Source: CAD feature listing. Evaluate the final solid. Frame: model axes, mm. Face numbers are marked on the shaded views. A direction names the side the tool comes from. Give positions to 0.01 mm unless a question says otherwise; leave off trailing zeros. Order: outer loops, then holes, each group sorted by start corner. A loop starts at its lowest first (then second) coordinate and runs counter-clockwise, first axis right, second up. Notation, with made-up numbers: (10, 18) - (14, 18) arc R34 ccw to (14, 49) - close; hole circle Ø11 at (22, 44.25). An arc over 180 degrees is marked (long way). Write each question's results on one line, items separated by ' | '. Start each with the question number.
Item 1: Line query: line 1 along X through (y, z) = (-12.75, 5.25); line 2 along Z through (x, y) = (12, -10); line 3 along Y through (x, z) = (5, 1.15). Output: solid intervals per line, ascending.
Item 2: Mould query, pull axis X, two halves, no side actions, for the marked faces 4, 5 and 6. Classes: released by +X, released by -X, zero draft, split by the parting line, or undercut.
Item 3: Section D-D on x = 31.5. Output: boundary loops of the cut face in (y, z) (1 decimal), and give its area (3 significant figures).
Item 4: Section A-A on x = 4.5. Output: boundary loops of the cut face in (y, z).
Item 5: Contact query for flat-ended pins moving along their axis: pin 1 Ø6 at (x, y) = (6, -4) entering from -Z; pin 2 Ø1.3 at (x, y) = (14.5, -6.5) entering from +Z; pin 3 Ø1.4 at (x, z) = (23, 12.5) entering from +Y; pin 4 Ø2 at (x, z) = (23.5, 11) entering from -Y. Output: stop coordinate, or through.
Item 6: Set-up query: the marked faces 1, 2 and 3. Return all of +Z, -Z, +X, -X, +Y, -Y with unobstructed straight access to the full face (end or side cutting, diameter ignored); none if empty.
Item 7: Section B-B on y = -10. State how many separate pieces and enclosed holes the cut face has, and give its area (3 significant figures).
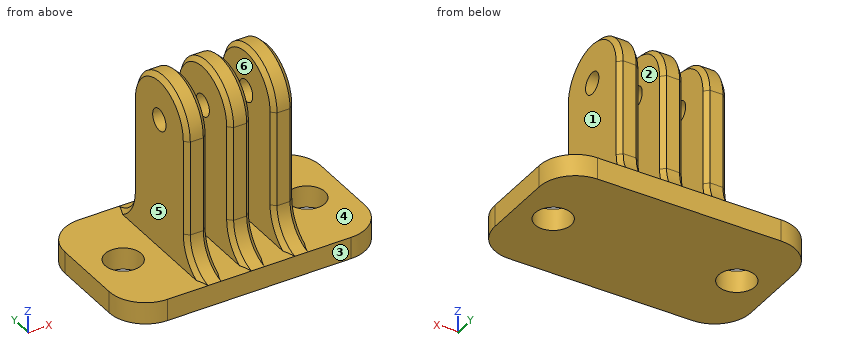
```python
from build123d import *

# Parameters (mm, degrees)
SKETCH_1_W             = 35.4
SKETCH_1_H             = 20
SKETCH_1_R             = 2.5
EXTRUDE_1_DEPTH        = 3
EXTRUDE_START          = -10
SKETCH_3_R             = 1.5
EXTRUDE_2_DEPTH        = 3
PATTERN_LINEAR_1_COUNT = 3
PATTERN_LINEAR_1_PITCH = 6
FILLET_1_R             = 5
CHAMFER_1_SIZE         = 0.6


with BuildPart() as part:
    # 草图1 → 凸台-拉伸1 (new body)
    with BuildSketch(Plane.XY):
        with Locations((17.7, -10)):
            Rectangle(SKETCH_1_W, SKETCH_1_H)
        with Locations((5, -10)):
            Circle(SKETCH_1_R, mode=Mode.SUBTRACT)
        with Locations((30.4, -10)):
            Circle(SKETCH_1_R, mode=Mode.SUBTRACT)
    extrude(amount=EXTRUDE_1_DEPTH)

    # 草图3 → 凸台-拉伸2 (add)
    with BuildSketch(Plane.ZY.offset(EXTRUDE_START)):
        with BuildLine():
            Line((3, -4), (21, -4))
            ThreePointArc((21, -4), (27, -10), (21, -16))
            Line((21, -16), (3, -16))
            Line((3, -16), (3, -4))
        make_face()
        with Locations(Location((21, -10, 0), (0, 0, 270))):
            Circle(SKETCH_3_R, mode=Mode.SUBTRACT)
    extrude_2 = extrude(amount=-EXTRUDE_2_DEPTH)

    # 阵列(线性)1: 凸台-拉伸2 ×3
    with Locations(*[(i * PATTERN_LINEAR_1_PITCH, 0, 0) for i in range(1, PATTERN_LINEAR_1_COUNT)]):
        add(extrude_2)

    # 圆角1
    # the kernel refuses this fillet: 5 mm, written as the material it adds along each edge
    with BuildSketch(Plane(origin=(10, -16, 3), x_dir=(0, -1.0, 1.572297847473644e-12), z_dir=(1, 0, 0)), Plane(origin=(16, -16, 3), x_dir=(0, -1.0, 1.572297847473644e-12), z_dir=(1, 0, 0)), Plane(origin=(22, -16, 3), x_dir=(0, -1.0, 1.572297847473644e-12), z_dir=(1, 0, 0))) as fillet_1_piece_1:
        with BuildLine():
            CenterArc((5, -4.898979486), FILLET_1_R, 101.536959033, 78.463040967)
            Line((0, -4.898979486), (0, 0))
            Line((0, 0), (4, 0))
        make_face()
    extrude(amount=3)
    with BuildSketch(Plane(origin=(-2.247448714, -16, 3), x_dir=(0, -1.0, 1.572297847473644e-12), z_dir=(1, 0, 0))) as fillet_1_piece_2_section:
        with BuildLine():
            CenterArc((5, -4.898979486), FILLET_1_R, 101.536959033, 78.463040967)
            Line((0, -4.898979486), (0, 0))
            Line((0, 0), (4, 0))
        make_face()
    fillet_1_piece_2 = extrude(amount=27.494897428, mode=Mode.PRIVATE)
    fillet_1_piece_2 = split(fillet_1_piece_2, bisect_by=Plane(origin=(16, -16, 3), z_dir=(1, 0, 0)), keep=Keep.TOP, mode=Mode.PRIVATE)
    fillet_1_piece_2 = split(fillet_1_piece_2, bisect_by=Plane(origin=(19, -16, 3), z_dir=(-1, 0, 0)), keep=Keep.TOP, mode=Mode.PRIVATE)
    add(fillet_1_piece_2)
    with BuildSketch(Plane(origin=(-2.247448714, -16, 3), x_dir=(0, -1.0, 1.572297847473644e-12), z_dir=(1, 0, 0))) as fillet_1_piece_3_section:
        with BuildLine():
            CenterArc((5, -4.898979486), FILLET_1_R, 101.536959033, 78.463040967)
            Line((0, -4.898979486), (0, 0))
            Line((0, 0), (4, 0))
        make_face()
    fillet_1_piece_3 = extrude(amount=27.494897428, mode=Mode.PRIVATE)
    fillet_1_piece_3 = split(fillet_1_piece_3, bisect_by=Plane(origin=(25, -16, 3), z_dir=(-1, 0, 0)), keep=Keep.TOP, mode=Mode.PRIVATE)
    fillet_1_piece_3 = split(fillet_1_piece_3, bisect_by=Plane(origin=(22, -16, 3), z_dir=(1, 0, 0)), keep=Keep.TOP, mode=Mode.PRIVATE)
    add(fillet_1_piece_3)
    with BuildSketch(Plane(origin=(10, -4, 3), x_dir=(0, 1.0, 1.568078999980068e-12), z_dir=(1, 0, 0)), Plane(origin=(16, -4, 3), x_dir=(0, 1.0, 1.568078999980068e-12), z_dir=(1, 0, 0)), Plane(origin=(22, -4, 3), x_dir=(0, 1.0, 1.568078999980068e-12), z_dir=(1, 0, 0))) as fillet_1_piece_4:
        with BuildLine():
            CenterArc((5, 4.898979486), FILLET_1_R, 180, 78.463040967)
            Line((0, 4.898979486), (0, 0))
            Line((0, 0), (4, 0))
        make_face()
    extrude(amount=3)
    with BuildSketch(Plane(origin=(-2.247448714, -4, 3), x_dir=(0, 1.0, 1.568078999980068e-12), z_dir=(1, 0, 0))) as fillet_1_piece_5_section:
        with BuildLine():
            CenterArc((5, 4.898979486), FILLET_1_R, 180, 78.463040967)
            Line((0, 4.898979486), (0, 0))
            Line((0, 0), (4, 0))
        make_face()
    fillet_1_piece_5 = extrude(amount=27.494897428, mode=Mode.PRIVATE)
    fillet_1_piece_5 = split(fillet_1_piece_5, bisect_by=Plane(origin=(16, -4, 3), z_dir=(1, 0, 0)), keep=Keep.TOP, mode=Mode.PRIVATE)
    fillet_1_piece_5 = split(fillet_1_piece_5, bisect_by=Plane(origin=(19, -4, 3), z_dir=(-1, 0, 0)), keep=Keep.TOP, mode=Mode.PRIVATE)
    add(fillet_1_piece_5)
    with BuildSketch(Plane(origin=(-2.247448714, -4, 3), x_dir=(0, 1.0, 1.568078999980068e-12), z_dir=(1, 0, 0))) as fillet_1_piece_6_section:
        with BuildLine():
            CenterArc((5, 4.898979486), FILLET_1_R, 180, 78.463040967)
            Line((0, 4.898979486), (0, 0))
            Line((0, 0), (4, 0))
        make_face()
    fillet_1_piece_6 = extrude(amount=27.494897428, mode=Mode.PRIVATE)
    fillet_1_piece_6 = split(fillet_1_piece_6, bisect_by=Plane(origin=(25, -4, 3), z_dir=(-1, 0, 0)), keep=Keep.TOP, mode=Mode.PRIVATE)
    fillet_1_piece_6 = split(fillet_1_piece_6, bisect_by=Plane(origin=(22, -4, 3), z_dir=(1, 0, 0)), keep=Keep.TOP, mode=Mode.PRIVATE)
    add(fillet_1_piece_6)
    with BuildSketch(Plane(origin=(3.752551286, -16, 3), x_dir=(0, -1.0, 1.572297847473644e-12), z_dir=(1, 0, 0))) as fillet_1_piece_7_section:
        with BuildLine():
            CenterArc((5, -4.898979486), FILLET_1_R, 101.536959033, 78.463040967)
            Line((0, -4.898979486), (0, 0))
            Line((0, 0), (4, 0))
        make_face()
    fillet_1_piece_7 = extrude(amount=27.494897428, mode=Mode.PRIVATE)
    fillet_1_piece_7 = split(fillet_1_piece_7, bisect_by=Plane(origin=(10, -16, 3), z_dir=(1, 0, 0)), keep=Keep.TOP, mode=Mode.PRIVATE)
    fillet_1_piece_7 = split(fillet_1_piece_7, bisect_by=Plane(origin=(13, -16, 3), z_dir=(-1, 0, 0)), keep=Keep.TOP, mode=Mode.PRIVATE)
    add(fillet_1_piece_7)
    with BuildSketch(Plane(origin=(3.752551286, -16, 3), x_dir=(0, -1.0, 1.572297847473644e-12), z_dir=(1, 0, 0))) as fillet_1_piece_8_section:
        with BuildLine():
            CenterArc((5, -4.898979486), FILLET_1_R, 101.536959033, 78.463040967)
            Line((0, -4.898979486), (0, 0))
            Line((0, 0), (4, 0))
        make_face()
    fillet_1_piece_8 = extrude(amount=27.494897428, mode=Mode.PRIVATE)
    fillet_1_piece_8 = split(fillet_1_piece_8, bisect_by=Plane(origin=(25, -16, 3), z_dir=(-1, 0, 0)), keep=Keep.TOP, mode=Mode.PRIVATE)
    fillet_1_piece_8 = split(fillet_1_piece_8, bisect_by=Plane(origin=(22, -16, 3), z_dir=(1, 0, 0)), keep=Keep.TOP, mode=Mode.PRIVATE)
    add(fillet_1_piece_8)
    with BuildSketch(Plane(origin=(3.752551286, -4, 3), x_dir=(0, 1.0, 1.568078999980068e-12), z_dir=(1, 0, 0))) as fillet_1_piece_9_section:
        with BuildLine():
            CenterArc((5, 4.898979486), FILLET_1_R, 180, 78.463040967)
            Line((0, 4.898979486), (0, 0))
            Line((0, 0), (4, 0))
        make_face()
    fillet_1_piece_9 = extrude(amount=27.494897428, mode=Mode.PRIVATE)
    fillet_1_piece_9 = split(fillet_1_piece_9, bisect_by=Plane(origin=(10, -4, 3), z_dir=(1, 0, 0)), keep=Keep.TOP, mode=Mode.PRIVATE)
    fillet_1_piece_9 = split(fillet_1_piece_9, bisect_by=Plane(origin=(13, -4, 3), z_dir=(-1, 0, 0)), keep=Keep.TOP, mode=Mode.PRIVATE)
    add(fillet_1_piece_9)
    with BuildSketch(Plane(origin=(3.752551286, -4, 3), x_dir=(0, 1.0, 1.568078999980068e-12), z_dir=(1, 0, 0))) as fillet_1_piece_10_section:
        with BuildLine():
            CenterArc((5, 4.898979486), FILLET_1_R, 180, 78.463040967)
            Line((0, 4.898979486), (0, 0))
            Line((0, 0), (4, 0))
        make_face()
    fillet_1_piece_10 = extrude(amount=27.494897428, mode=Mode.PRIVATE)
    fillet_1_piece_10 = split(fillet_1_piece_10, bisect_by=Plane(origin=(25, -4, 3), z_dir=(-1, 0, 0)), keep=Keep.TOP, mode=Mode.PRIVATE)
    fillet_1_piece_10 = split(fillet_1_piece_10, bisect_by=Plane(origin=(22, -4, 3), z_dir=(1, 0, 0)), keep=Keep.TOP, mode=Mode.PRIVATE)
    add(fillet_1_piece_10)
    with BuildSketch(Plane(origin=(9.752551286, -16, 3), x_dir=(0, -1.0, 1.572297847473644e-12), z_dir=(1, 0, 0))) as fillet_1_piece_11_section:
        with BuildLine():
            CenterArc((5, -4.898979486), FILLET_1_R, 101.536959033, 78.463040967)
            Line((0, -4.898979486), (0, 0))
            Line((0, 0), (4, 0))
        make_face()
    fillet_1_piece_11 = extrude(amount=27.494897428, mode=Mode.PRIVATE)
    fillet_1_piece_11 = split(fillet_1_piece_11, bisect_by=Plane(origin=(10, -16, 3), z_dir=(1, 0, 0)), keep=Keep.TOP, mode=Mode.PRIVATE)
    fillet_1_piece_11 = split(fillet_1_piece_11, bisect_by=Plane(origin=(13, -16, 3), z_dir=(-1, 0, 0)), keep=Keep.TOP, mode=Mode.PRIVATE)
    add(fillet_1_piece_11)
    with BuildSketch(Plane(origin=(9.752551286, -16, 3), x_dir=(0, -1.0, 1.572297847473644e-12), z_dir=(1, 0, 0))) as fillet_1_piece_12_section:
        with BuildLine():
            CenterArc((5, -4.898979486), FILLET_1_R, 101.536959033, 78.463040967)
            Line((0, -4.898979486), (0, 0))
            Line((0, 0), (4, 0))
        make_face()
    fillet_1_piece_12 = extrude(amount=27.494897428, mode=Mode.PRIVATE)
    fillet_1_piece_12 = split(fillet_1_piece_12, bisect_by=Plane(origin=(16, -16, 3), z_dir=(1, 0, 0)), keep=Keep.TOP, mode=Mode.PRIVATE)
    fillet_1_piece_12 = split(fillet_1_piece_12, bisect_by=Plane(origin=(19, -16, 3), z_dir=(-1, 0, 0)), keep=Keep.TOP, mode=Mode.PRIVATE)
    add(fillet_1_piece_12)
    with BuildSketch(Plane(origin=(9.752551286, -4, 3), x_dir=(0, 1.0, 1.568078999980068e-12), z_dir=(1, 0, 0))) as fillet_1_piece_13_section:
        with BuildLine():
            CenterArc((5, 4.898979486), FILLET_1_R, 180, 78.463040967)
            Line((0, 4.898979486), (0, 0))
            Line((0, 0), (4, 0))
        make_face()
    fillet_1_piece_13 = extrude(amount=27.494897428, mode=Mode.PRIVATE)
    fillet_1_piece_13 = split(fillet_1_piece_13, bisect_by=Plane(origin=(10, -4, 3), z_dir=(1, 0, 0)), keep=Keep.TOP, mode=Mode.PRIVATE)
    fillet_1_piece_13 = split(fillet_1_piece_13, bisect_by=Plane(origin=(13, -4, 3), z_dir=(-1, 0, 0)), keep=Keep.TOP, mode=Mode.PRIVATE)
    add(fillet_1_piece_13)
    with BuildSketch(Plane(origin=(9.752551286, -4, 3), x_dir=(0, 1.0, 1.568078999980068e-12), z_dir=(1, 0, 0))) as fillet_1_piece_14_section:
        with BuildLine():
            CenterArc((5, 4.898979486), FILLET_1_R, 180, 78.463040967)
            Line((0, 4.898979486), (0, 0))
            Line((0, 0), (4, 0))
        make_face()
    fillet_1_piece_14 = extrude(amount=27.494897428, mode=Mode.PRIVATE)
    fillet_1_piece_14 = split(fillet_1_piece_14, bisect_by=Plane(origin=(16, -4, 3), z_dir=(1, 0, 0)), keep=Keep.TOP, mode=Mode.PRIVATE)
    fillet_1_piece_14 = split(fillet_1_piece_14, bisect_by=Plane(origin=(19, -4, 3), z_dir=(-1, 0, 0)), keep=Keep.TOP, mode=Mode.PRIVATE)
    add(fillet_1_piece_14)
    # the kernel refuses this fillet: 5 mm, written as the material it takes off along each edge
    with BuildSketch(Plane(origin=(0, 0, -12.5), x_dir=(1, 0, 0), z_dir=(0, 0, 1)), Plane(origin=(35.4, -20, -12.5), x_dir=(-1, 0, 0), z_dir=(0, 0, 1))) as fillet_1_2_piece_1:
        with BuildLine():
            CenterArc((FILLET_1_R, -FILLET_1_R), FILLET_1_R, 90, 90)
            Line((0, -FILLET_1_R), (0, 0))
            Line((0, 0), (FILLET_1_R, 0))
        make_face()
    extrude(amount=28, mode=Mode.SUBTRACT)
    with BuildSketch(Plane(origin=(35.4, 0, -12.5), x_dir=(-1, 0, 0), z_dir=(0, 0, 1)), Plane(origin=(0, -20, -12.5), x_dir=(1, 0, 0), z_dir=(0, 0, 1))) as fillet_1_2_piece_2:
        with BuildLine():
            CenterArc((FILLET_1_R, FILLET_1_R), FILLET_1_R, 180, 90)
            Line((0, FILLET_1_R), (0, 0))
            Line((0, 0), (FILLET_1_R, 0))
        make_face()
    extrude(amount=28, mode=Mode.SUBTRACT)

    # 倒角1
    chamfer_1_edges = [part.edges().sort_by_distance(p)[0] for p in [
        (13, -4, 14.449489743),
        (13, -10, 27),
        (10, -10, 27),
        (10, -4, 14.449489743),
        (19, -4, 14.449489743),
        (19, -10, 27),
        (16, -10, 27),
        (16, -4, 14.449489743),
        (25, -4, 14.449489743),
        (25, -10, 27),
        (22, -10, 27),
        (22, -4, 14.449489743),
        (10, -16, 14.449489743),
        (13, -16, 14.449489743),
        (16, -16, 14.449489743),
        (19, -16, 14.449489743),
        (22, -16, 14.449489743),
        (25, -16, 14.449489743),
        (10, -17.127016654, 4.736701825),
        (13, -17.127016654, 4.736701825),
        (16, -17.127016654, 4.736701825),
        (19, -17.127016654, 4.736701825),
        (22, -17.127016654, 4.736701825),
        (25, -17.127016654, 4.736701825),
        (10, -2.872983346, 4.736701825),
        (13, -2.872983346, 4.736701825),
        (16, -2.872983346, 4.736701825),
        (19, -2.872983346, 4.736701825),
        (22, -2.872983346, 4.736701825),
        (25, -2.872983346, 4.736701825),
    ]]
    chamfer(chamfer_1_edges, length=CHAMFER_1_SIZE)


solid = part.part
```
Evaluation:
1) line 1: x = 10 to 13, 16 to 19, 22 to 25 | line 2: z = 0 to 19.5, 22.5 to 27 | line 3: y = -20 to -12.5, -7.5 to 0
2) face 4: zero draft | face 5: released by -X | face 6: undercut
3) outline: (-19.9, 0) - (-12.2, 0) - (-12.2, 3) - (-19.9, 3) - close; (-7.8, 0) - (-0.1, 0) - (-0.1, 3) - (-7.8, 3) - close | area: 45.8 mm^2
4) outline: (-19.97, 0) - (-12.45, 0) - (-12.45, 3) - (-19.97, 3) - close; (-7.55, 0) - (-0.03, 0) - (-0.03, 3) - (-7.55, 3) - close
5) pin 1: stops at z = 0 | pin 2: stops at z = 3 | pin 3: stops at y = -4 | pin 4: stops at y = -16
6) face 1: +Z, +X, +Y, -Y | face 2: +Z, +Y, -Y | face 3: +Z, -Z, +X, -X, -Y
7) separate pieces: 6 | enclosed holes: 0 | area: 264 mm^2
